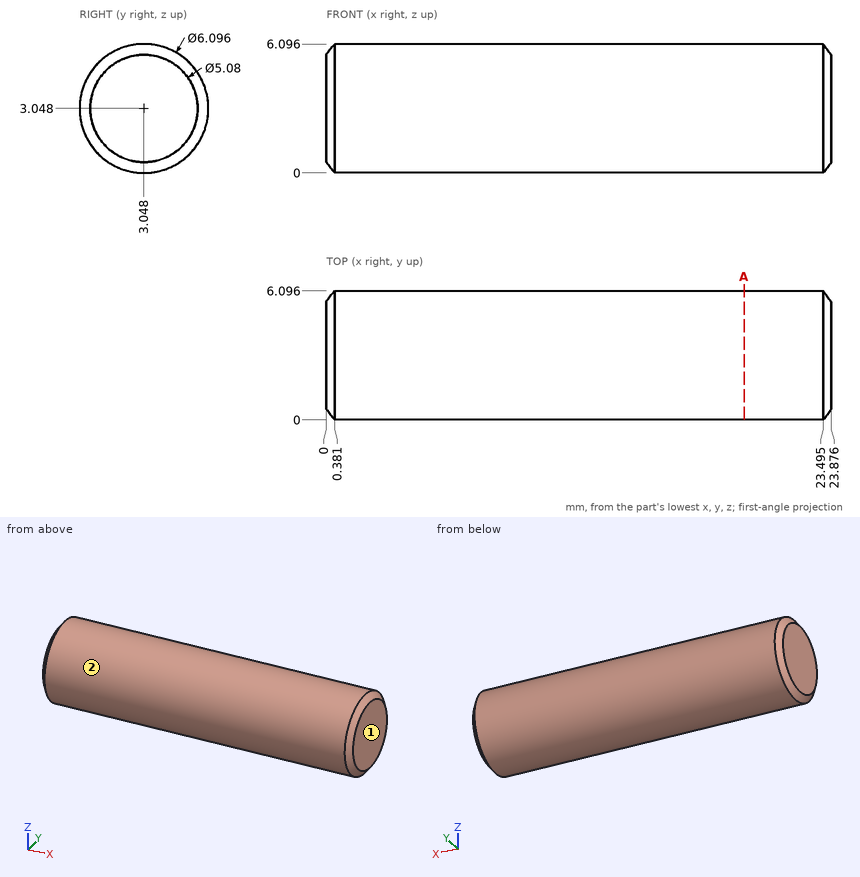
Verification items for this drawing (mm, ordinates from the low corner). Give positions to 0.01 mm unless a question says otherwise; leave off trailing zeros. Loops run counter-clockwise (first coordinate to the right, second up) from the corner with the lowest first, then second, coordinate; pieces in that order, holes last.
1. Go/stop test with flat-tipped pins: P1, Ø2, axis at x = 15, z = 4, coming from the +Y side; P2, Ø1, axis at x = 18, z = 4.5, coming from the -Y side. Record where each tip stops, or that it passes through.
Derived:
P1: stops at y = 6.1
P2: stops at y = 0.15
2. Release check for a two-part mould opening along Z. For the marked faces 1 and 2 record: +Z half, -Z half, draft (parallel to the pull), parting line (faces both ways), or undercut.
Derived:
face 1: draft
face 2: parting line
3. Cross-section at A-A on x = 19.75. Record the cut outline in (y, z), and give its area (3 significant figures).
Derived:
outline: circle Ø6.1 at (3.05, 3.05)
area: 29.2 mm2
4. Material ranges on probe 1 along Y at (x, z) = (11.25, 1.75); probe 2 along X at (y, z) = (4.5, 5.25); probe 3 along Z at (x, y) = (12, 5.75), recorded low to high.
Derived:
probe 1: y = 0.29 to 5.81
probe 2: x = 0.07 to 23.8
probe 3: z = 1.64 to 4.46
